Answer from the drawing. Dimensions are ordinates in mm from the lowest x, y and z of the part. Round coordinates to 2 decimals unless told otherwise and drop trailing zeros. Loops run counter-clockwise (first coordinate to the right, second up) from the corner with the lowest first, then second, coordinate; pieces in that order, holes last. Notation, with made-up numbers: (24, 63.5) - (68, 63.5) arc R23 ccw to (68, 86.5) - close; hole circle Ø11 at (79.5, 24.25). An arc over 180 degrees is marked (long way). Answer as CSV lines item,"result".
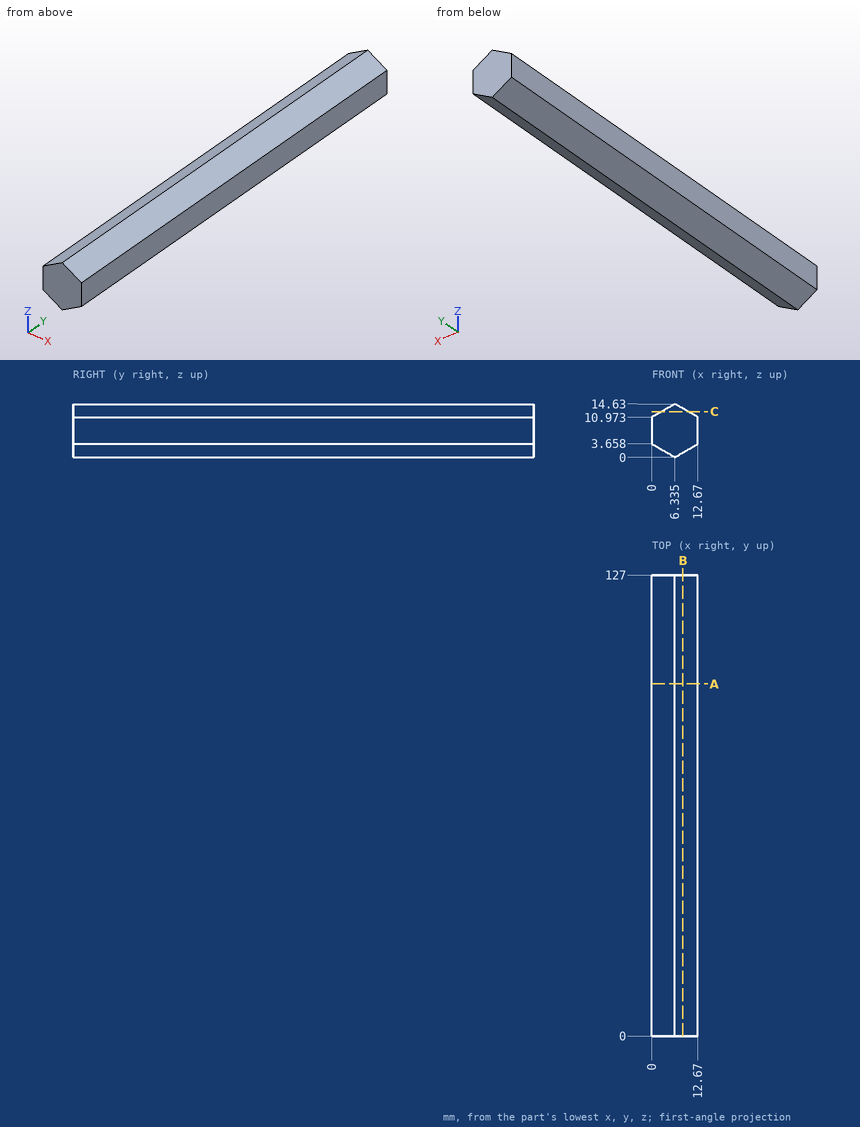
1) A cutting plane is placed at B-B, the plane x = 8.5. Determine the outline of the cut face in (y, z), plus the area to 3 significant figures.
Entries:
outline,"(0, 1.25) - (127, 1.25) - (127, 13.38) - (0, 13.38) - close"
area,"1,540 mm^2"
2) A cutting plane is placed at C-C, the plane z = 12.5. Determine the outline of the cut face in (x, y) (1 decimal), plus the area to 3 significant figures.
Entries:
outline,"(2.6, 0) - (10, 0) - (10, 127) - (2.6, 127) - close"
area,"937 mm^2"
3) Find the intervals of material crossed by line 1 (X direction, y = 36.5, z = 11.75) (1 decimal); line 2 (Z direction, x = 8.75, y = 113.5) (1 decimal); line 3 (Z direction, x = 4, y = 20.5), in increasing order.
Entries:
line 1,"x = 1.3 to 11.3"
line 2,"z = 1.4 to 13.2"
line 3,"z = 1.35 to 13.28"
4) A cutting plane is placed at A-A, the plane y = 97. Determine the outline of the cut face in (x, z) (1 decimal).
Entries:
outline,"(0, 3.7) - (6.3, 0) - (12.7, 3.7) - (12.7, 11) - (6.3, 14.6) - (0, 11) - close"
5) Each of these flat-tipped pins is pushed along its axis until it touches: P1, Ø1, axis at x = 4, y = 13.5, coming from the +Z side; P2, Ø6, axis at x = 2.5, y = 88, coming from the -Z side. Where does it stop, or does it pass through?
Entries:
P1,"stops at z = 13.57"
P2,"stops at z = 0.48"
